from build123d import *

# Parameters (mm, degrees)
ESQUISSE2_W        = 246
ESQUISSE2_H        = 96
ESQUISSE2_W_2      = 205
ESQUISSE2_H_2      = 54.8
BOSS_EXTRU_1_DEPTH = 10
CONG_1_R           = 8
ESQUISSE3_W        = 205
ESQUISSE3_H        = 54.8
BOSS_EXTRU_2_DEPTH = 2


with BuildPart() as part:
    # Esquisse2 → Boss.-Extru.1 (new body)
    with BuildSketch(Plane.XY):
        with Locations((123, 48)):
            Rectangle(ESQUISSE2_W, ESQUISSE2_H)
        with Locations((123, 48)):
            Rectangle(ESQUISSE2_W_2, ESQUISSE2_H_2, mode=Mode.SUBTRACT)
    extrude(amount=BOSS_EXTRU_1_DEPTH)

    # Congé1
    cong_1_edges = [part.edges().sort_by_distance(p)[0] for p in [
        (0, 96, 5),
        (246, 96, 5),
        (246, 0, 5),
        (0, 0, 5),
    ]]
    fillet(cong_1_edges, radius=CONG_1_R)

    # Esquisse3 → Boss.-Extru.2 (add)
    with BuildSketch(Plane(origin=(0, 0, 0), x_dir=(-1, 0, 0), z_dir=(0, 0, -1))):
        with Locations((-123, 48)):
            Rectangle(ESQUISSE3_W, ESQUISSE3_H)
    extrude(amount=-BOSS_EXTRU_2_DEPTH)


solid = part.part
Model file for the job. Use its own axes, mm. A direction names the side the tool comes from. Coordinates: 2 decimals unless noted, no trailing zeros. Write each loop counter-clockwise with the first axis right and the second up, starting at its lowest first coordinate (ties: lowest second). Pieces come first, ordered by that corner, then holes. Notation, with made-up numbers: (11, 77) -> (48, 77) arc R28 cw to (48, 97) -> close; hole circle Ø11 at (-3.75, 68.25). An arc over 180 degrees is marked (long way). One line per item, written item: value. Start each with the question number.
1) Flat gauge pins, fed straight in: pin 1 Ø12 at (x, y) = (145, 54) entering from +Z; pin 2 Ø12 at (x, y) = (33, 71.5) entering from +Z. Where does each tip first touch, or does it go through?
2) Probe probe 1 along X at (y, z) = (32, 2.5); probe 2 along Y at (x, z) = (84, 5.75); probe 3 along Z at (x, y) = (132, 45). List the from-to ranges inside material, lowest first.
3) Slice it at A-A on x = 132. Write the cut outline in (y, z).
4) Slice it at C-C on y = 24. Write the cut outline in (x, z), then the cut area to 3 significant figures.
5) Slice it at B-B on z = 6. Write the cut outline in (x, y).
6) Which spindle directions (+Z, -Z, +X, -X, +Y, -Y) get a long thin tool onto all of the face, cutting with end or side? Do faces 1 (the face through (0, 47, 5)), 2 (the face through (20.5, 48, 6)). Say none if no direction does.
7) Pull direction Y, two halves, no side cores. Call faces 3 (the face through (122, 75.4, 6)), 4 (the face through (243.594, 2.281, 5.07)), 5 (the face through (246, 47, 5)): +Y half, -Y half, draft (parallel to the pull), parting line (faces both ways), or undercut.
Answers follow:
1. pin 1: z = 2
1. pin 2: z = 10
2. probe 1: 0 to 20.5, 225.5 to 246
2. probe 2: 0 to 20.6, 75.4 to 96
2. probe 3: 0 to 2
3. outline: (0, 0) -> (96, 0) -> (96, 10) -> (75.4, 10) -> (75.4, 2) -> (20.6, 2) -> (20.6, 10) -> (0, 10) -> close
4. outline: (0, 0) -> (246, 0) -> (246, 10) -> (225.5, 10) -> (225.5, 2) -> (20.5, 2) -> (20.5, 10) -> (0, 10) -> close
4. area: 820 mm2
5. outline: (0, 8) arc R8 ccw to (8, 0) -> (238, 0) arc R8 ccw to (246, 8) -> (246, 88) arc R8 ccw to (238, 96) -> (8, 96) arc R8 ccw to (0, 88) -> close; hole (20.5, 20.6) -> (225.5, 20.6) -> (225.5, 75.4) -> (20.5, 75.4) -> close
6. face 1: +Z, -Z, -X, +Y, -Y
6. face 2: +Z
7. face 3: undercut
7. face 4: -Y half
7. face 5: draft
